For this review, take the finished solid that the model builds, in its own axes (mm). A direction names the side the tool comes from. Coordinates: 2 decimals unless noted, no trailing zeros. Order: outer loops, then holes, each group sorted by start corner. A loop starts at its lowest first (then second) coordinate and runs counter-clockwise, first axis right, second up.
Autodesk Inventor part; units mm, degrees
ref_plane "YZ Plane" through (0, 0, 0) normal (1, 0, 0) x (0, 1, 0)
ref_plane "XZ Plane" through (0, 0, 0) normal (0, 1, 0) x (-1, 0, 0)
ref_plane "XY Plane" through (0, 0, 0) normal (0, 0, 1) x (1, 0, 0)
sketch "Sketch1" plane through (0, 0, 0) normal (0, 0, 1) x (1, 0, 0)
  line L0 (-179, 3) -> (-179, 30)
  line L1 (-179, 30) -> (-199, 30)
  line L2 (-274, 126) -> (-244, 126)
  line L3 (-274, 126) -> (-274, 70)
  arc A0 (-239.9746, 21.3454) -> (-199, 0) centre (-199, 50) ccw
  line L4 (-274, 70) -> (-239.9746, 21.3454)
  line L5 (0, 0) -> (-199, 0) construction
  line L6 (-244, 126) -> (-244, 79.4492)
  line L7 (-244, 79.4492) -> (-215.3898, 38.5382)
  arc A1 (-215.3898, 38.5382) -> (-199, 30) centre (-199, 50) ccw
  line L8 (-179, 3) -> (-199, 3)
  line L9 (-199, 3) -> (-199, 0)
  line L10 (0, -31.2197) -> (0, 152.2033) construction
  line L11 (-239.9746, 21.3454) -> (-215.3898, 38.5382) construction
  dimension "d3" = 50
  dimension "d4" = 123
  dimension "d5" = 65
  dimension "d6" = 30
  dimension "d11" = 30
  dimension "d22" = 199
  dimension "d23" = 20
  dimension "d32" = 3
  dimension "d42" = 27
  dimension "d44" = 70
revolve "Revolution1" add sketch "Sketch1" angle 360 about axis through (0, -10, 0) along (0, 1, 0)
chamfer "Chamfer1" distance 5 angle 45 1 edges at (179, 30, 0)
properties material "Polyethylene, Low Density"
1. The part is to be moulded in two halves that separate along Z. For faces 4 (the face through (184, 126, -161)), 5 (the face through (47.08, 41.097, -212.015)), 6 (the face through (52.483, 24.389, -236.346)), say which applies: +Z half, -Z half, draft (parallel to the pull), parting line (faces both ways), or undercut.
Answer below:
face 4: draft
face 5: undercut
face 6: parting line
2. Take a section at C-C, the plane y = 108.5. Give the boundary of the cut face in (x, z), plus the area to 3 significant figures.
Answer below:
outline: circle Ø548 at (0, 0); hole circle Ø488 at (0, 0)
area: 48,800 mm2
3. Clearance check with flat-ended pins moving along their axes: pin 1 Ø1.5 at (y, z) = (83, 134.5) entering from +X; pin 2 Ø1.5 at (x, y) = (92, 30) entering from +Z; pin 3 Ø6 at (y, z) = (113, 145) entering from -X. State where each tip first meets the part, or that it passes through.
Answer below:
pin 1: stops at x = 239.14
pin 2: stops at z = 228.82
pin 3: stops at x = -234.33
4. Machinability: for faces 1 (the face through (193.63, 102.4, 148.47)), 2 (the face through (-82.598, 14.154, -158.804)), 3 (the face through (163, 3, 75)), which of the approach directions +Z, -Z, +X, -X, +Y, -Y give a long, thin tool a straight path to every point of the face, cutting with its end or side? Answer none if there is none.
Answer below:
face 1: +Y
face 2: +Y, -Y
face 3: -Y
5. Take a section at B-B, the plane z = 0. Give the boundary of the cut face in (x, y), plus the area to 3 significant figures.
Answer below:
outline: (-274, 70) - (-239.97, 21.35) arc R50 ccw to (-199, 0) - (-199, 3) - (-179, 3) - (-179, 25) - (-184, 30) - (-199, 30) arc R20 cw to (-215.39, 38.54) - (-244, 79.45) - (-244, 126) - (-274, 126) - close; (179, 3) - (199, 3) - (199, 0) arc R50 ccw to (239.97, 21.35) - (274, 70) - (274, 126) - (244, 126) - (244, 79.45) - (215.39, 38.54) arc R20 cw to (199, 30) - (184, 30) - (179, 25) - close
area: 9,430 mm2
6. To check wall thickness, follow L1, parallel to Z at x = 0, y = 97.5; L2, parallel to Z at x = 190.5, y = 95.5; L3, parallel to X at y = 107.5, z = 189. State the ranges of each line that lie inside material, in increasing order.
Answer below:
L1: z = -274 to -244, 244 to 274
L2: z = -196.94 to -152.47, 152.47 to 196.94
L3: x = -198.38 to -154.32, 154.32 to 198.38
7. Take a section at D-D, the plane y = 13. Give the boundary of the cut face in (x, z), plus the area to 3 significant figures.
Answer below:
outline: circle Ø465.26 at (0, 0); hole circle Ø358 at (0, 0)
area: 69,400 mm2
8. Take a section at A-A, the plane x = 0. Give the boundary of the cut face in (y, z), plus the area to 3 significant figures.
Answer below:
outline: (0, -199) arc R50 ccw to (21.35, -239.97) - (70, -274) - (126, -274) - (126, -244) - (79.45, -244) - (38.54, -215.39) arc R20 cw to (30, -199) - (30, -184) - (25, -179) - (3, -179) - (3, -199) - close; (0, 199) - (3, 199) - (3, 179) - (25, 179) - (30, 184) - (30, 199) arc R20 cw to (38.54, 215.39) - (79.45, 244) - (126, 244) - (126, 274) - (70, 274) - (21.35, 239.97) arc R50 ccw to start
area: 9,430 mm2
